Build history of the part. All positions in model axes, mm. Give positions to 0.01 mm unless a question says otherwise; leave off trailing zeros. Loops run counter-clockwise (first coordinate to the right, second up) from the corner with the lowest first, then second, coordinate; pieces in that order, holes last. Notation, with made-up numbers: (12, 20) -> (20, 20) arc R34 cw to (20, 58) -> close; hole circle Ø5 at (58.25, 43.25). An arc over 180 degrees is marked (long way). Answer in a Markdown table with one row per item. Add a question column.
Autodesk Inventor part; units mm, degrees
ref_plane "YZ Plane" through (0, 0, 0) normal (1, 0, 0) x (0, 1, 0)
ref_plane "XZ Plane" through (0, 0, 0) normal (0, 1, 0) x (-1, 0, 0)
ref_plane "XY Plane" through (0, 0, 0) normal (0, 0, 1) x (1, 0, 0)
sketch "Sketch1" plane through (0, 0, 0) normal (0, 1, 0) x (-1, 0, 0)
  line L0 (0, -5.3526) -> (-4.6355, -2.6763)
  line L1 (-4.6355, -2.6763) -> (-4.6355, 2.6763)
  line L2 (-4.6355, 2.6763) -> (0, 5.3526)
  line L3 (0, 5.3526) -> (4.6355, 2.6763)
  line L4 (4.6355, 2.6763) -> (4.6355, -2.6763)
  line L5 (4.6355, -2.6763) -> (0, -5.3526)
  point P0 (0, 0)
  point P1 (0, 0)
  dimension "d0" = 9.271
extrude "Extrusion1" add sketch "Sketch1" along normal blind 101.6
sketch "Sketch2" plane through (4.6355, 0, 2.6763) normal (0.5, 0, 0.866) x (0.866, 0, -0.5)
  line L0 (-5.3526, 101.6) -> (0, 101.6)
  line L1 (0, 0) -> (-5.3526, 0)
  point P0 (-2.6763, 0)
  point P1 (-2.7496, 17.399)
  point P2 (-2.7496, 84.201)
  dimension "d3" = 17.399
  dimension "d4" = 17.399
hole "Hole1" at (2.2543, 17.399, 4.0511) at (2.2543, 84.201, 4.0511) direction (-0.5, 0, -0.866) diameter 5.1054 end through all
equation "\"printingError\" = 0.254"
equation "\"depthForHexBolt\" = 17.399"
properties part number "3_8_plasticPipe"
(1) Wall check: line 1 along Y through (x, z) = (0.25, 0.5); line 2 along Y through (x, z) = (-4, -2); line 3 along Z through (x, y) = (1.25, 74). Give the ranges that are in metal, low to high. Write a range as from..to.
(2) Two-plate mould, pull along X, no slides. Class faces 1 (the flat face through (0, 101.6, 0)), 2 (the flat face through (-2.29, 50.09, 4.03)), 3 (the cylindrical face through (0.751, 81.843, -0.508)): released by +X, released by -X, zero draft, split by the parting line, or undercut.
(3) Saw through at C-C, the plane z = 1.75. State how many separate pieces and enclosed holes the cut face has, then the cut area to 3 significant figures.
(4) Saw through at B-B, the plane y = 95.5. List the corners of the cut face in (x, z), then the cut area to 3 significant figures.
(5) Saw through at A-A, the plane y = 16. List the corners of the cut face in (x, z).
Worked answers:
| question | item | result |
|---|---|---|
| 1 | line 1 | 0..14.85, 19.95..81.65, 86.75..101.6 |
| 1 | line 2 | 0..16.5, 18.29..83.31, 85.1..101.6 |
| 1 | line 3 | -4.63..4.63 |
| 2 | face 1 | zero draft |
| 2 | face 2 | released by -X |
| 2 | face 3 | undercut |
| 3 | separate pieces | 1 |
| 3 | enclosed holes | 2 |
| 3 | area | 895 mm^2 |
| 4 | outline | (-4.64, -2.68) -> (0, -5.35) -> (4.64, -2.68) -> (4.64, 2.68) -> (0, 5.35) -> (-4.64, 2.68) -> close |
| 4 | area | 74.4 mm^2 |
| 5 | outline | (-4.64, -2.68) -> (-4.23, -2.91) -> (0.41, 5.12) -> (0, 5.35) -> (-4.64, 2.68) -> close; (-0.53, -5.05) -> (0, -5.35) -> (4.64, -2.68) -> (4.64, 2.68) -> (4.1, 2.98) -> close |
